The model under review builds one solid part; all positions refer to its coordinate system, in mm. A direction names the side the tool comes from. Give positions to 0.01 mm unless a question says otherwise; leave off trailing zeros. Write each loop counter-clockwise with the first axis right and the second up, starting at its lowest first coordinate (ties: lowest second). Pieces come first, ordered by that corner, then holes. Notation, with made-up numbers: (0.25, 51) - (4.25, 51) arc R35 ccw to (4.25, 84) - close; hole circle Ø4 at (38.5, -34.75). An arc over 180 degrees is marked (long way). Write item = value, one per line.
```python
from build123d import *

# Parameters (mm, degrees)
SKETCH1_R           = 46.5
SKETCH1_R_2         = 36
BOSS_EXTRUDE1_DEPTH = 28.7
SKETCH2_R           = 2.25
CUT_EXTRUDE1_DEPTH  = 72.750888496
CUT_EXTRUDE2_START  = -5.5
SKETCH3_R           = 37.5
SKETCH3_R_2         = 36
CUT_EXTRUDE2_DEPTH  = 5.5


with BuildPart() as part:
    # Sketch1 → Boss-Extrude1 (new body)
    with BuildSketch(Plane(origin=(0, 0, 0), x_dir=(1, 0, 0), z_dir=(0, 1, 0))):
        with Locations(Location((0, 0, 0), (0, 0, 270))):
            Circle(SKETCH1_R)
        with Locations(Location((0, 0, 0), (0, 0, 270))):
            Circle(SKETCH1_R_2, mode=Mode.SUBTRACT)
    extrude(amount=BOSS_EXTRUDE1_DEPTH)

    # Sketch2 → Cut-Extrude1 (cut, through all)
    with BuildSketch(Plane(origin=(0, 28.7, 0), x_dir=(1, 0, 0), z_dir=(0, 1, 0))):
        with Locations(Location((0, 41, 0), (0, 0, 270))):
            Circle(SKETCH2_R)
        with Locations(Location((28.991378029, 28.991378029, 0), (0, 0, 270))):
            Circle(SKETCH2_R)
        with Locations(Location((41, 0, 0), (0, 0, 270))):
            Circle(SKETCH2_R)
        with Locations(Location((28.991378029, -28.991378029, 0), (0, 0, 270))):
            Circle(SKETCH2_R)
        with Locations(Location((0, -41, 0), (0, 0, 270))):
            Circle(SKETCH2_R)
        with Locations(Location((-28.991378029, -28.991378029, 0), (0, 0, 270))):
            Circle(SKETCH2_R)
        with Locations(Location((-41, 0, 0), (0, 0, 270))):
            Circle(SKETCH2_R)
        with Locations(Location((-28.991378029, 28.991378029, 0), (0, 0, 270))):
            Circle(SKETCH2_R)
    extrude(amount=-CUT_EXTRUDE1_DEPTH, mode=Mode.SUBTRACT)

    # Sketch3 → Cut-Extrude2 (cut)
    with BuildSketch(Plane(origin=(0, 28.7, 0), x_dir=(1, 0, 0), z_dir=(0, 1, 0)).offset(CUT_EXTRUDE2_START)):
        with Locations(Location((0, 0, 0), (0, 0, 270))):
            Circle(SKETCH3_R)
        with Locations(Location((0, 0, 0), (0, 0, 270))):
            Circle(SKETCH3_R_2, mode=Mode.SUBTRACT)
    extrude(amount=CUT_EXTRUDE2_DEPTH, mode=Mode.SUBTRACT)


solid = part.part
```
1. Draft analysis for pull direction Z (two halves, no side actions). For faces 1 (the cylindrical face through (46.1, 14.1, -6.1)), 2 (the flat face through (-34, 0, -14)), 3 (the cylindrical face through (0.099, 14.551, -43.248)), 4 (the cylindrical face through (29.667, 14.551, 31.137)), state which applies: +Z half, -Z half, draft (parallel to the pull), parting line (faces both ways), or undercut.
Findings below:
face_1 = parting line
face_2 = draft
face_3 = undercut
face_4 = undercut
2. For line 1 (X direction, y = 7, z = 0); line 2 (X direction, y = 27.5, z = 0); line 3 (Z direction, x = -2, y = 19.5), list the stretches that pass through material, from the lowest coordinate up. Write a range as from..to.
Findings below:
line_1 = -46.5..-43.25, -38.75..-36, 36..38.75, 43.25..46.5
line_2 = -46.5..-43.25, -38.75..-37.5, 37.5..38.75, 43.25..46.5
line_3 = -46.46..-42.03, -39.97..-35.94, 35.94..39.97, 42.03..46.46
3. Take a section at A-A on z = 0. Give the boundary of the cut face in (x, y).
Findings below:
outline = (-46.5, 0) - (-43.25, 0) - (-43.25, 28.7) - (-46.5, 28.7) - close; (-38.75, 0) - (-36, 0) - (-36, 23.2) - (-37.5, 23.2) - (-37.5, 28.7) - (-38.75, 28.7) - close; (36, 0) - (38.75, 0) - (38.75, 28.7) - (37.5, 28.7) - (37.5, 23.2) - (36, 23.2) - close; (43.25, 0) - (46.5, 0) - (46.5, 28.7) - (43.25, 28.7) - close
4. Insertion check: P1, Ø10, axis at x = 33.5, y = 5.5, coming from the +Z side; P2, Ø4, axis at x = -28.99, z = -28.99, coming from the +Y side; P3, Ø12, axis at y = 11.5, z = -11, coming from the -X side; P4, Ø6, axis at x = 28.99, z = -28.99, coming from the +Y side. Each pin has a flat end and moves straight along its axis. Give the tip position at first contact, or say it passes through.
Findings below:
P1 = 36.74
P2 = through
P3 = -46.23
P4 = 28.7
5. Take a section at C-C on z = -41. Give the boundary of the cut face in (x, y).
Findings below:
outline = (-21.94, 0) - (-2.25, 0) - (-2.25, 28.7) - (-21.94, 28.7) - close; (2.25, 0) - (21.94, 0) - (21.94, 28.7) - (2.25, 28.7) - close
6. Take a section at D-D on x = -16.5. Give the boundary of the cut face in (y, z), and give its area (3 significant figures).
Findings below:
outline = (0, -43.47) - (28.7, -43.47) - (28.7, -33.67) - (23.2, -33.67) - (23.2, -32) - (0, -32) - close; (0, 32) - (23.2, 32) - (23.2, 33.67) - (28.7, 33.67) - (28.7, 43.47) - (0, 43.47) - close
area = 640 mm²
7. Machinability: for faces 5 (the cylindrical face through (-28.32, 14.55, 31.14)), 6 (the flat face through (34, 23.2, -14)), which of the approach directions +Z, -Z, +X, -X, +Y, -Y give a long, thin tool a straight path to every point of the face, cutting with its end or side? Answer none if there is none.
Findings below:
face_5 = +Y, -Y
face_6 = +Y
8. Take a section at B-B on x = 0. Give the boundary of the cut face in (y, z), and give its area (3 significant figures).
Findings below:
outline = (0, -46.5) - (28.7, -46.5) - (28.7, -43.25) - (0, -43.25) - close; (0, -38.75) - (28.7, -38.75) - (28.7, -37.5) - (23.2, -37.5) - (23.2, -36) - (0, -36) - close; (0, 36) - (23.2, 36) - (23.2, 37.5) - (28.7, 37.5) - (28.7, 38.75) - (0, 38.75) - close; (0, 43.25) - (28.7, 43.25) - (28.7, 46.5) - (0, 46.5) - close
area = 328 mm²
